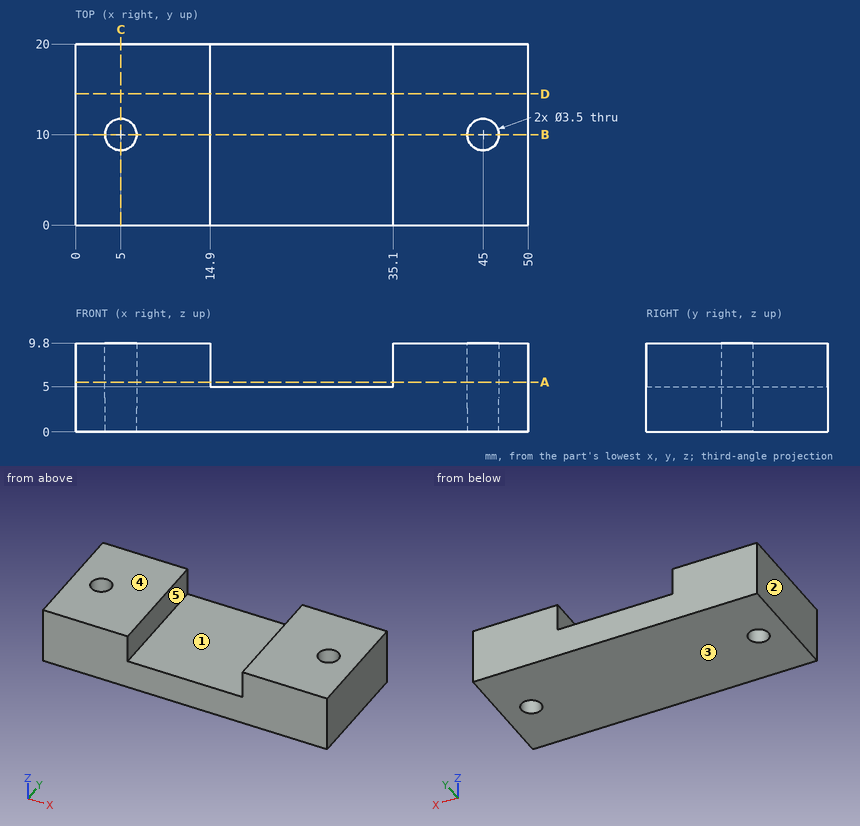
Job drawing, mm, ordinate dimensions from the low corner. One solid piece. A direction names the side the tool comes from. Give positions to 0.01 mm unless a question says otherwise; leave off trailing zeros. Write each loop counter-clockwise with the first axis right and the second up, starting at its lowest first coordinate (ties: lowest second). Pieces come first, ordered by that corner, then holes. Notation, with made-up numbers: (58, 84.25) -> (91, 84.25) arc R14 cw to (91, 109.25) -> close; hole circle Ø3 at (-19.75, 69). An arc over 180 degrees is marked (long way). Return JSON: item names as keys, results as strings.
Item 1: Tool access for the marked faces 4 and 5: list every direction of +Z, -Z, +X, -X, +Y, -Y with a clear straight run to the whole face (end or side of a thin tool).
Answer below:
{"face 4": "+Z, +X, -X, +Y, -Y", "face 5": "+Z, +Y, -Y"}
Item 2: Two-plate mould, pull along X, no slides. Class the marked faces 1, 2 and 3: +X half, -X half, draft (parallel to the pull), parting line (faces both ways), or undercut.
Answer below:
{"face 1": "undercut", "face 2": "-X half", "face 3": "draft"}
Item 3: Band-saw the part on B-B (y = 10). List the corners of the cut face in (x, z), then the cut area to 3 significant figures.
Answer below:
{"outline": "(0, 0) -> (3.25, 0) -> (3.25, 9.8) -> (0, 9.8) -> close; (6.75, 0) -> (43.25, 0) -> (43.25, 9.8) -> (35.1, 9.8) -> (35.1, 5) -> (14.9, 5) -> (14.9, 9.8) -> (6.75, 9.8) -> close; (46.75, 0) -> (50, 0) -> (50, 9.8) -> (46.75, 9.8) -> close", "area": "324 mm2"}
Item 4: Band-saw the part on D-D (y = 14.5). List the corners of the cut face in (x, z).
Answer below:
{"outline": "(0, 0) -> (50, 0) -> (50, 9.8) -> (35.1, 9.8) -> (35.1, 5) -> (14.9, 5) -> (14.9, 9.8) -> (0, 9.8) -> close"}
Item 5: Drill centre lines: probe 1 along X at (y, z) = (10, 7); probe 2 along X at (y, z) = (18.75, 7.5); probe 3 along Y at (x, z) = (45, 7.75). Where is each one in solid material? Low to high.
Answer below:
{"probe 1": "x = 0 to 3.25, 6.75 to 14.9, 35.1 to 43.25, 46.75 to 50", "probe 2": "x = 0 to 14.9, 35.1 to 50", "probe 3": "y = 0 to 8.25, 11.75 to 20"}
Item 6: Band-saw the part on A-A (z = 5.5). List the corners of the cut face in (x, y), then the cut area to 3 significant figures.
Answer below:
{"outline": "(0, 0) -> (14.9, 0) -> (14.9, 20) -> (0, 20) -> close; (35.1, 0) -> (50, 0) -> (50, 20) -> (35.1, 20) -> close; hole circle Ø3.5 at (5, 10); hole circle Ø3.5 at (45, 10)", "area": "577 mm2"}
Item 7: Band-saw the part on C-C (x = 5). List the corners of the cut face in (y, z), then the cut area to 3 significant figures.
Answer below:
{"outline": "(0, 0) -> (8.25, 0) -> (8.25, 9.8) -> (0, 9.8) -> close; (11.75, 0) -> (20, 0) -> (20, 9.8) -> (11.75, 9.8) -> close", "area": "162 mm2"}
Item 8: Drop flat-ended pins along their axis: pin 1 (1 mm diameter, centred on x = 22, z = 1.5, fed in from -Y); pin 2 (10 mm diameter, centred on x = 23.5, y = 9.5, fed in from +Z); pin 3 (3 mm diameter, centred on x = 5, y = 10, fed in from -Z). Give the stop position or say it passes through.
Answer below:
{"pin 1": "stops at y = 0", "pin 2": "stops at z = 5", "pin 3": "passes through"}
